from build123d import *

# Parameters (mm, degrees)
F0_R     = 1.9685
F1_DEPTH = 3.4544
F2_W     = 1.9558
F2_H     = 0.9525
F2_W_2   = 1.9431
F3_DEPTH = 16.7142
F5_DEPTH = 12.7
F6_R     = 0.254


with BuildPart() as f1:
    # F0 (on Top) → F1 (new body)
    with BuildSketch(Plane.XY):
        with BuildLine():
            Line((8.3566, 5.9309), (-3.7846, 5.9309))
            ThreePointArc((-3.7846, 5.9309), (-7.0174922036, 4.5917922036), (-8.3566, 1.3589))
            Line((-8.3566, 1.3589), (-8.3566, -1.3589))
            ThreePointArc((-8.3566, -1.3589), (-7.0174922036, -4.5917922036), (-3.7846, -5.9309))
            Line((-3.7846, -5.9309), (2.413, -5.9309))
            Line((2.413, -5.9309), (2.413, -3.4671))
            Line((2.413, -3.4671), (8.3566, -3.4671))
            Line((8.3566, -3.4671), (8.3566, 5.9309))
        make_face()
        with Locations((-0.4318, 0)):
            Circle(F0_R, mode=Mode.SUBTRACT)
    extrude(amount=F1_DEPTH)

    # F2 (on face) → F3 (cut, through all)
    with BuildSketch(Plane.YZ.offset(8.3566)):
        with Locations((4.953, 2.97815)):
            Rectangle(F2_W, F2_H)
        with Locations((-4.95935, 2.97815)):
            Rectangle(F2_W_2, F2_H)
    extrude(amount=-F3_DEPTH, mode=Mode.SUBTRACT)

    # F4 (on Front) → F5 (cut, symmetric)
    with BuildSketch(Plane.XZ):
        with BuildLine():
            Line((8.3566, 1.3984937485), (8.3566, 3.4544))
            Line((8.3566, 3.4544), (5.985548453, 3.4544))
            ThreePointArc((5.985548453, 3.4544), (7.3183634134, 2.596313693), (8.3566, 1.3984937485))
        make_face()
    extrude(amount=F5_DEPTH, both=True, mode=Mode.SUBTRACT)

    # F6
    f6_edges = [f1.edges().sort_by_distance(p)[0] for p in [
        (-2.556099, -3.9878, 3.4544),
        (-0.774271, 3.9751, 3.4544),
        (-2.556099, -3.9878, 2.5019),
        (-0.054799, 3.9751, 2.5019),
    ]]
    fillet(f6_edges, radius=F6_R)

    # F7 (on Front) → F8 (revolve, cut)
    with BuildSketch(Plane.XZ):
        Polygon((-2.4003, 0.6604), (-2.7815821178, 0), (-0.4318, 0), (-0.4318, 0.6604), align=None)
    revolve(axis=Axis((-0.4318, 0, 0.3302), (0, 0, 1)), mode=Mode.SUBTRACT)


solid = f1.part
Design review of the part built by this model. Coordinates are the model's own, in mm. A direction names the side the tool comes from. Round coordinates to 2 decimals unless told otherwise and drop trailing zeros. Write each loop counter-clockwise with the first axis right and the second up, starting at its lowest first coordinate (ties: lowest second). Pieces come first, ordered by that corner, then holes. Notation, with made-up numbers: (-9, 43.25) - (7, 43.25) arc R24 cw to (7, 67.25) - close; hole circle Ø2 at (1.25, -14). An arc over 180 degrees is marked (long way). Return JSON: item names as keys, results as strings. Group by question number.
Item 1: Insertion check: P1, Ø0.9, axis at x = 0.5, y = 5, coming from the +Z side; P2, Ø1, axis at x = 5.5, z = 1.5, coming from the -Y side; P3, Ø0.7, axis at y = -4.5, z = 2.5, coming from the +X side. Each pin has a flat end and moves straight along its axis. Give the tip position at first contact, or say it passes through.
Item 2: Machinability: for faces 5 (the face through (0, 5, 2.502)), 6 (the face through (-2, -5, 2.502)), 7 (the face through (5, -3.467, 2)), which of the approach directions +Z, -Z, +X, -X, +Y, -Y give a long, thin tool a straight path to every point of the face, cutting with its end or side? Answer none if there is none.
Item 3: For probe 1 along Y at (x, z) = (-0.5, 2.8); probe 2 along Y at (x, z) = (7.25, 2.45); probe 3 along X at (y, z) = (1, 1.5), list the stretches that pass through material, from the lowest coordinate up. Write a range as [from, to].
Item 4: We need section B-B on x = 5.25. Write out the cut boundary in (y, z).
Item 5: We need section C-C on z = 0.9. Write out the cut boundary in (x, y), and give its area (3 significant figures).
Item 6: We need section D-D on z = 2.3. Write out the cut boundary in (x, y), and give its area (3 significant figures).
Item 7: We need section A-A on y = 0. Write out the cut boundary in (x, z), and give its area (3 significant figures).
Item 8: The part is to be moulded in two halves that separate along Y. For faces 1 (the face through (2, 1, 0)), 2 (the face through (-6.98, 4.63, 1.32)), 3 (the face through (-0.86, -1.92, 2.04)), 4 (the face through (-7.05, -4.56, 1.7)), say which applies: pulls with the +Y half, pulls with the -Y half, needs draft (parallel to the pull), parting line crosses it, or undercut.
Model answer:
{
 "1": {"P1": "stops at z = 2.5", "P2": "stops at y = -3.47", "P3": "stops at x = 2.41"},
 "2": {"face 5": "+Z, +X, -X, +Y", "face 6": "+Z, +X, -X, -Y", "face 7": "+Z, -Z, +X, -Y"},
 "3": {"probe 1": "y = [-3.99, -1.97], [1.97, 3.98]", "probe 2": "y = [-3.47, 5.93]", "probe 3": "x = [-8.36, -2.13], [1.26, 8.29]"},
 "4": {"outline": "(-3.47, 0) - (5.93, 0) - (5.93, 2.5) - (4.23, 2.5) arc R0.25 cw to (3.98, 2.76) - (3.98, 3.2) arc R0.25 ccw to (3.72, 3.45) - (-3.47, 3.45) - close"},
 "5": {"outline": "(-8.36, -1.36) arc R4.57 ccw to (-3.78, -5.93) - (2.41, -5.93) - (2.41, -3.47) - (8.36, -3.47) - (8.36, 5.93) - (-3.78, 5.93) arc R4.57 ccw to (-8.36, 1.36) - close; hole circle Ø3.94 at (-0.43, 0)", "area": "162 mm²"},
 "6": {"outline": "(-8.36, -1.36) arc R4.57 ccw to (-3.78, -5.93) - (2.41, -5.93) - (2.41, -3.47) - (7.63, -3.47) - (7.63, 5.93) - (-3.78, 5.93) arc R4.57 ccw to (-8.36, 1.36) - close; hole circle Ø3.94 at (-0.43, 0)", "area": "156 mm²"},
 "7": {"outline": "(-8.36, 0) - (-2.78, 0) - (-2.4, 0.66) - (-2.4, 3.45) - (-8.36, 3.45) - close; (1.54, 0.66) - (1.92, 0) - (8.36, 0) - (8.36, 1.4) arc R5.59 ccw to (5.99, 3.45) - (1.54, 3.45) - close", "area": "41.9 mm²"},
 "8": {"face 1": "needs draft", "face 2": "pulls with the +Y half", "face 3": "undercut", "face 4": "pulls with the -Y half"}
}
